Design review of the part shown in the three views and the two pictorial views. Dimensions are in mm from the part's minimum x, y and z. Give positions to 0.01 mm unless a question says otherwise; leave off trailing zeros. Order: outer loops, then holes, each group sorted by start corner. A loop starts at its lowest first (then second) coordinate and runs counter-clockwise, first axis right, second up. Notation, with made-up numbers: (78, 4) -> (127, 4) arc R26 cw to (127, 31) -> close; hole circle Ø6 at (-27, 9). An arc over 180 degrees is marked (long way). Answer in a Markdown table with one row per item. Add a question column.
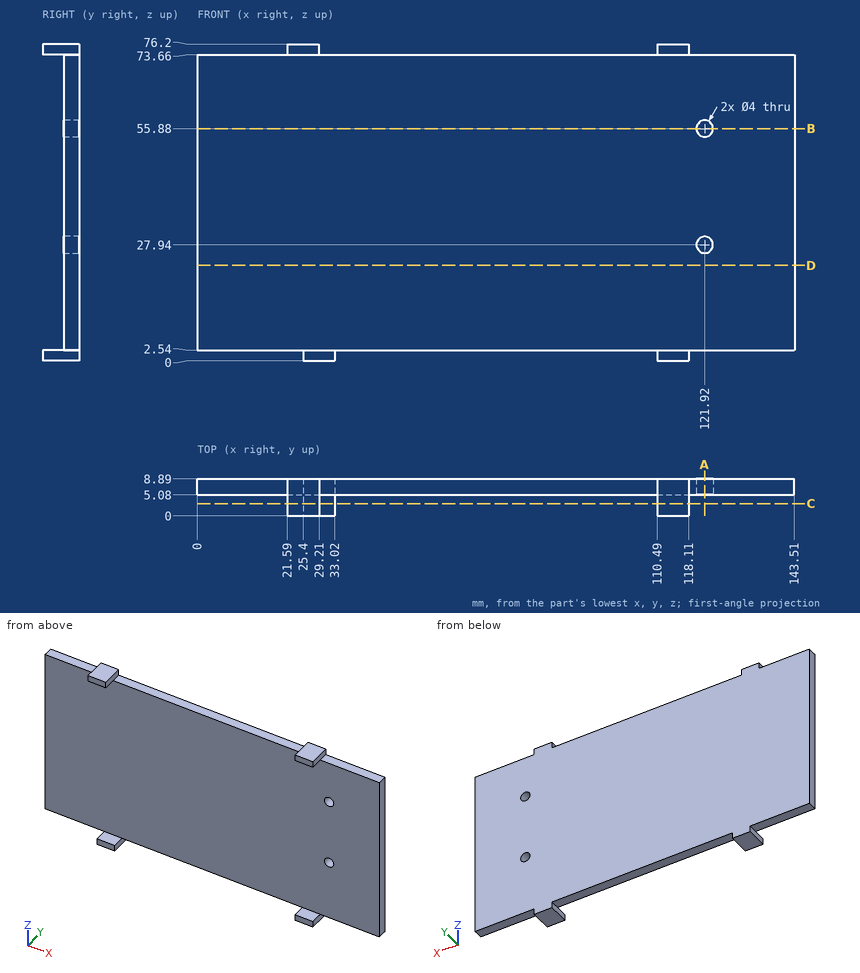
1) Add section D-D, the plane z = 23. Write out the cut boundary in (x, y).
2) Clearance check with flat-ended pins moving along their axes: P1, Ø1.9, axis at x = 13.5, y = 6.5, coming from the -Z side; P2, Ø0.8, axis at y = 6.5, z = 75, coming from the +X side; P3, Ø2, axis at y = 6.5, z = 75.5, coming from the -X side. State where each tip first meets the part, or that it passes through.
3) Add section A-A, the plane x = 121.92. Write out the cut boundary in (y, z), and give its area (3 significant figures).
4) For L1, parallel to X at y = 7.9, z = 55.88; L2, parallel to Y at x = 117.5, z = 53; L3, parallel to Z at x = 42, y = 6.25, list the stretches that pass through material, from the lowest coordinate up.
5) Add section C-C, the plane y = 3. Write out the cut boundary in (x, z), and give its area (3 significant figures).
6) Add section B-B, the plane z = 55.88. Write out the cut boundary in (x, y), and give its area (3 significant figures).
Verdict:
| question | item | result |
|---|---|---|
| 1 | outline | (0, 5.08) -> (143.51, 5.08) -> (143.51, 8.89) -> (0, 8.89) -> close |
| 2 | P1 | stops at z = 2.54 |
| 2 | P2 | stops at x = 118.11 |
| 2 | P3 | stops at x = 21.59 |
| 3 | outline | (5.08, 2.54) -> (8.89, 2.54) -> (8.89, 25.94) -> (5.08, 25.94) -> close; (5.08, 29.94) -> (8.89, 29.94) -> (8.89, 53.88) -> (5.08, 53.88) -> close; (5.08, 57.88) -> (8.89, 57.88) -> (8.89, 73.66) -> (5.08, 73.66) -> close |
| 3 | area | 240 mm2 |
| 4 | L1 | x = 0 to 119.92, 123.92 to 143.51 |
| 4 | L2 | y = 5.08 to 8.89 |
| 4 | L3 | z = 2.54 to 73.66 |
| 5 | outline | (21.59, 73.66) -> (29.21, 73.66) -> (29.21, 76.2) -> (21.59, 76.2) -> close; (25.4, 0) -> (33.02, 0) -> (33.02, 2.54) -> (25.4, 2.54) -> close; (110.49, 0) -> (118.11, 0) -> (118.11, 2.54) -> (110.49, 2.54) -> close; (110.49, 73.66) -> (118.11, 73.66) -> (118.11, 76.2) -> (110.49, 76.2) -> close |
| 5 | area | 77.4 mm2 |
| 6 | outline | (0, 5.08) -> (119.92, 5.08) -> (119.92, 8.89) -> (0, 8.89) -> close; (123.92, 5.08) -> (143.51, 5.08) -> (143.51, 8.89) -> (123.92, 8.89) -> close |
| 6 | area | 532 mm2 |
